```python
from build123d import *

# Parameters (mm, degrees)
SKETCH_W        = 12
SKETCH_H        = 18.5
SKETCH_R        = 2.5
PAD_DEPTH       = 7
SKETCH001_W     = 12
SKETCH001_H     = 6.5
POCKET_DEPTH    = 2
SKETCH002_R     = 1.5
POCKET001_DEPTH = 5.001
SKETCH003_R     = 4
PAD001_DEPTH    = 3
SKETCH004_R     = 2.5
POCKET002_DEPTH = 5
FILLET_R        = 4
CHAMFER_SIZE    = 1


with BuildPart() as part:
    # Sketch → Pad (new body)
    with BuildSketch(Plane.XY):
        with Locations((0, -3.25)):
            Rectangle(SKETCH_W, SKETCH_H)
        Circle(SKETCH_R, mode=Mode.SUBTRACT)
    extrude(amount=PAD_DEPTH)

    # Sketch001 (on Face6 of Pad) → Pocket (cut)
    with BuildSketch(Plane(origin=(0, 0, 0), x_dir=(1, 0, 0), z_dir=(0, 0, -1))):
        with Locations((0, 8)):
            Rectangle(SKETCH001_W, SKETCH001_H)
    extrude(amount=-POCKET_DEPTH, mode=Mode.SUBTRACT)

    # Sketch002 (on Face7 of Pocket) → Pocket001 (cut, through all)
    with BuildSketch(Plane(origin=(0, 0, 2), x_dir=(1, 0, 0), z_dir=(0, 0, -1))):
        with Locations((0, 8)):
            Circle(SKETCH002_R)
    extrude(amount=-POCKET001_DEPTH, mode=Mode.SUBTRACT)

    # Sketch003 (on Face7 of Pad) → Pad001 (join)
    with BuildSketch(Plane.XY.offset(7)):
        Circle(SKETCH003_R)
    extrude(amount=PAD001_DEPTH)

    # Sketch004 (on Face15 of Pad001) → Pocket002 (cut)
    with BuildSketch(Plane.XY.offset(10)):
        Circle(SKETCH004_R)
    extrude(amount=-POCKET002_DEPTH, mode=Mode.SUBTRACT)

    # Fillet
    fillet_edges = [part.edges().sort_by_distance(p)[0] for p in [
        (6, 6, 3.5),
        (-6, 6, 3.5),
    ]]
    fillet(fillet_edges, radius=FILLET_R)

    # Chamfer
    chamfer_edges = [part.edges().sort_by_distance(p)[0] for p in [
        (-2.5, 0, 0),
    ]]
    chamfer(chamfer_edges, length=CHAMFER_SIZE)


solid = part.part
```
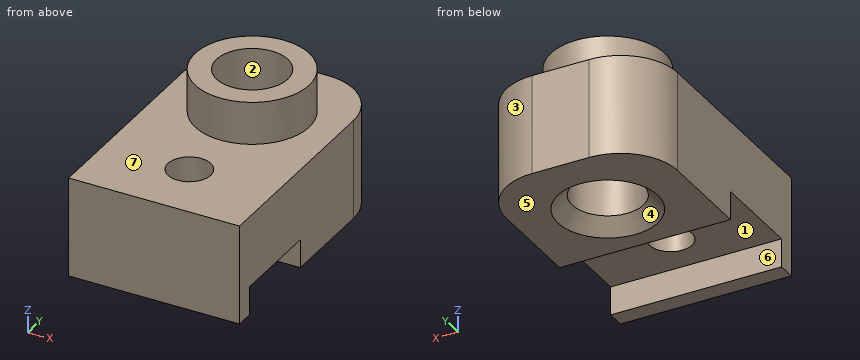
Geometry: final body of the model. Coordinates: model frame, mm. Face numbers are marked on the shaded views. A direction names the side the tool comes from. Give positions to 0.01 mm unless a question says otherwise; leave off trailing zeros. Loops run counter-clockwise (first coordinate to the right, second up) from the corner with the lowest first, then second, coordinate; pieces in that order, holes last. Notation, with made-up numbers: (43, 84) -> (89, 84) arc R26 cw to (89, 101) -> close; hole circle Ø7 at (32, 16.5). An arc over 180 degrees is marked (long way). Use CSV: the item, a comma, the result in double quotes.
(1) Ray query, line 1 along Y through (x, z) = (0, 3.25); line 2 along X through (y, z) = (-8, 4.05); line 3 along Y through (x, z) = (0.5, 6.5). Return the intervals inside material, ascending. Write a range as [from, to].
From the geometry:
line 1,"[-12.5, -9.5], [-6.5, -2.5], [2.5, 6]"
line 2,"[-6, -1.5], [1.5, 6]"
line 3,"[-12.5, -9.41], [-6.59, -2.45], [2.45, 6]"
(2) Cut plane D-D (y = -8). Output: boundary loops of the cut face in (x, z).
From the geometry:
outline,"(-6, 2) -> (-1.5, 2) -> (-1.5, 7) -> (-6, 7) -> close; (1.5, 2) -> (6, 2) -> (6, 7) -> (1.5, 7) -> close"
(3) Pull-direction query (X, two-part tool) for the marked faces 1, 2, 3 and 4; classes: released by +X, released by -X, zero draft, split by the parting line, or undercut.
From the geometry:
face 1,"zero draft"
face 2,"undercut"
face 3,"released by +X"
face 4,"undercut"
(4) Access query for the marked faces 5, 6 and 7. Directions: +Z, -Z, +X, -X, +Y, -Y. A direction counts if a zero-diameter tool reaches every point of the face in a straight line with its end or side. Return the directions, or none.
From the geometry:
face 5,"-Z, +X, -X, +Y, -Y"
face 6,"-Z, +X, -X"
face 7,"+Z"
(5) First-contact query: P1, Ø6.5, axis at x = 0, y = 0, coming from the -Z side; P2, Ø1, axis at x = 1.5, y = -9, coming from the -Z side; P3, Ø1.5, axis at x = -1, y = -9, coming from the +Z side. Flat tips, straight axial feed; report the tip coordinate or a pass-through.
From the geometry:
P1,"z = 0.25"
P2,"z = 2"
P3,"z = 7"
(6) Cut plane C-C (z = 5). Output: boundary loops of the cut face in (x, y), plus the area to 3 significant figures.
From the geometry:
outline,"(-6, -12.5) -> (6, -12.5) -> (6, 2) arc R4 ccw to (2, 6) -> (-2, 6) arc R4 ccw to (-6, 2) -> close; hole circle Ø5 at (0, 0); hole circle Ø3 at (0, -8)"
area,"188 mm^2"
(7) Cut plane B-B (x = 0). Output: boundary loops of the cut face in (y, z), plus the area to 3 significant figures.
From the geometry:
outline,"(-12.5, 0) -> (-11.25, 0) -> (-11.25, 2) -> (-9.5, 2) -> (-9.5, 7) -> (-12.5, 7) -> close; (-6.5, 2) -> (-4.75, 2) -> (-4.75, 0) -> (-3.5, 0) -> (-2.5, 1) -> (-2.5, 10) -> (-4, 10) -> (-4, 7) -> (-6.5, 7) -> close; (2.5, 1) -> (3.5, 0) -> (6, 0) -> (6, 7) -> (4, 7) -> (4, 10) -> (2.5, 10) -> close"
area,"74.5 mm^2"
(8) Cut plane A-A (y = 0). Output: boundary loops of the cut face in (x, z).
From the geometry:
outline,"(-6, 0) -> (-3.5, 0) -> (-2.5, 1) -> (-2.5, 10) -> (-4, 10) -> (-4, 7) -> (-6, 7) -> close; (2.5, 1) -> (3.5, 0) -> (6, 0) -> (6, 7) -> (4, 7) -> (4, 10) -> (2.5, 10) -> close"
